Design review of the part built by this model. Coordinates are the model's own, in mm. A direction names the side the tool comes from. Coordinates: 2 decimals unless noted, no trailing zeros. Loops run counter-clockwise (first coordinate to the right, second up) from the corner with the lowest first, then second, coordinate; pieces in that order, holes last. Notation, with made-up numbers: (46, 87.25) - (55, 87.25) arc R24 cw to (55, 98.25) - close; hole circle Ø3 at (37, 38). An arc over 180 degrees is marked (long way). Answer in a Markdown table with one row per item. Add a question column.
(1) Clearance check with flat-ended pins moving along their axes: pin 1 (1.6 mm diameter, centred on x = -10.5, z = -59, fed in from +Y); pin 2 (5 mm diameter, centred on x = 5.5, y = 15.5, fed in from +Z); pin 3 (10.5 mm diameter, centred on x = 0, z = 42, fed in from +Y); pin 4 (10 mm diameter, centred on x = 29, y = 23, fed in from -Z). State where each tip first meets the part, or that it passes through.
(2) We need section D-D, the plane y = 22.5. Write out the cut boundary in (x, z), plus the area to 3 significant figures.
(3) The part is to be moulded in two halves that separate along Z. For faces 3 (the face through (0, 1, -54)), 4 (the face through (39.24, 23.74, -39.2)), 5 (the face through (-39.26, 23.74, 39.2)), say which applies: released by +Z, released by -Z, zero draft, split by the parting line, or undercut.
(4) We need section C-C, the plane z = -45. Write out the cut boundary in (x, y), plus the area to 4 significant figures.
(5) We need section B-B, the plane y = 8.5. Write out the cut boundary in (x, z), plus the area to 4 significant figures.
(6) To check wall thickness, follow L1, parallel to X at y = 16.25, z = 34; L2, parallel to X at y = 1, z = -45; L3, parallel to Y at x = 39.35, z = 8. State the ranges of each line that lie inside material, in increasing order. Write a range as [from, to].
(7) We need section A-A, the plane x = 0. Write out the cut boundary in (y, z).
(8) For faces 1 (the face through (-38.5, 12, 1)), 2 (the face through (-39.26, 21.35, 5.23)), list the 3-axis set-ups (+Z, -Z, +X, -X, +Y, -Y) from which the entire face can be reached by the end or side of a thin tool; tool diameter is ignored.
from build123d import *

# Parameters (mm, degrees)
SKETCH1_W               = 80
SKETCH1_H               = 120
SKETCH1_R               = 4
SKETCH1_R_2             = 9
BOSS_EXTRUDE1_DEPTH     = 1.5
BOSS_EXTRUDE2_DEPTH     = 28
SKETCH2_3_W             = 77
SKETCH2_3_H             = 1.5
BOSS_EXTRUDE3_DEPTH     = 13
CUT_EXTRUDE1_DEPTH      = 78.911809118
CUT_EXTRUDE1_DEPTH_BACK = 78.911809118
SKETCH3_R               = 3
FILLET1_R               = 3


with BuildPart() as part:
    # Sketch1 → Boss-Extrude1 (new body)
    with BuildSketch(Plane(origin=(0, 0, 0), x_dir=(1, 0, 0), z_dir=(0, 1, 0))):
        Rectangle(SKETCH1_W, SKETCH1_H)
        with Locations(Location((0, -42, 0), (0, 0, 270))):
            Circle(SKETCH1_R, mode=Mode.SUBTRACT)
        with Locations(Location((0, 45, 0), (0, 0, 270))):
            Circle(SKETCH1_R_2, mode=Mode.SUBTRACT)
    extrude(amount=BOSS_EXTRUDE1_DEPTH)

    # Sketch2 → Boss-Extrude2 (add)
    with BuildSketch(Plane(origin=(0, 1.5, 0), x_dir=(1, 0, 0), z_dir=(0, 1, 0))):
        Polygon((-40, 60), (-40, 58.5), (-40, -60), (-38.5, -60), (-38.5, 58.5), (-38.5, 60), align=None)
        Polygon((38.5, 58.5), (38.5, -60), (40, -60), (40, 58.5), (40, 60), (38.5, 60), align=None)
    extrude(amount=BOSS_EXTRUDE2_DEPTH)

    # Sketch2_3 → Boss-Extrude3 (add)
    with BuildSketch(Plane(origin=(0, 1.5, 0), x_dir=(1, 0, 0), z_dir=(0, 1, 0))):
        with Locations((0, 59.25)):
            Rectangle(SKETCH2_3_W, SKETCH2_3_H)
    extrude(amount=BOSS_EXTRUDE3_DEPTH)

    # Sketch3 → Cut-Extrude1 (cut, two sides: drawn at the far end of the back side and taken through both)
    with BuildSketch(Plane(origin=(0, 0, 0), x_dir=(0, 0, -1), z_dir=(1, 0, 0)).offset(-CUT_EXTRUDE1_DEPTH_BACK)):
        with Locations((-8, 22.5)):
            Circle(SKETCH3_R)
        Polygon((20, 29.5), (60, 29.5), (60, 17.5), align=None)
        Polygon((-60, 17.5), (-20, 29.5), (-60, 29.5), align=None)
    extrude(amount=CUT_EXTRUDE1_DEPTH + CUT_EXTRUDE1_DEPTH_BACK, mode=Mode.SUBTRACT)

    # Fillet1
    fillet1_edges = [part.edges().sort_by_distance(p)[0] for p in [
        (39.25, 17.5, -60),
        (-39.25, 17.5, -60),
        (39.25, 17.5, 60),
        (-39.25, 17.5, 60),
    ]]
    fillet(fillet1_edges, radius=FILLET1_R)


solid = part.part
Responses:
| question | item | result |
|---|---|---|
| 1 | pin 1 | stops at y = 14.5 |
| 1 | pin 2 | stops at z = -58.5 |
| 1 | pin 3 | stops at y = 1.5 |
| 1 | pin 4 | passes through |
| 2 | outline | (-40, -43.33) - (-38.5, -43.33) - (-38.5, 5) - (-40, 5) - close; (-40, 11) - (-38.5, 11) - (-38.5, 43.33) - (-40, 43.33) - close; (38.5, -43.33) - (40, -43.33) - (40, 5) - (38.5, 5) - close; (38.5, 11) - (40, 11) - (40, 43.33) - (38.5, 43.33) - close |
| 2 | area | 242 mm2 |
| 3 | face 3 | undercut |
| 3 | face 4 | released by -Z |
| 3 | face 5 | released by +Z |
| 4 | outline | (-40, 0) - (-9, 0) - (-9, 1.5) - (-38.5, 1.5) - (-38.5, 22) - (-40, 22) - close; (9, 0) - (40, 0) - (40, 22) - (38.5, 22) - (38.5, 1.5) - (9, 1.5) - close |
| 4 | area | 154.5 mm2 |
| 5 | outline | (-40, -60) - (40, -60) - (40, 60) - (38.5, 60) - (38.5, -58.5) - (-38.5, -58.5) - (-38.5, 60) - (-40, 60) - close |
| 5 | area | 475.5 mm2 |
| 6 | L1 | x = [-40, -38.5], [38.5, 40] |
| 6 | L2 | x = [-40, -9], [9, 40] |
| 6 | L3 | y = [0, 19.5], [25.5, 29.5] |
| 7 | outline | (0, -60) - (14.5, -60) - (14.5, -58.5) - (1.5, -58.5) - (1.5, -54) - (0, -54) - close; (0, -36) - (1.5, -36) - (1.5, 38) - (0, 38) - close; (0, 46) - (1.5, 46) - (1.5, 60) - (0, 60) - close |
| 8 | face 1 | +Z, +Y |
| 8 | face 2 | +X, -X |
